Check sheet for the drawn part. Datum: minimum x, y, z corner. Units: mm. A direction names the side the tool comes from. Round coordinates to 2 decimals unless told otherwise and drop trailing zeros. Write each loop counter-clockwise with the first axis right and the second up, starting at its lowest first coordinate (ties: lowest second). Pieces come first, ordered by that corner, then holes. Notation, with made-up numbers: (17.5, -6) -> (46.5, -6) arc R15 ccw to (46.5, 6) -> close; hole circle Ø3 at (85, 4.25). An arc over 180 degrees is marked (long way). Use a Markdown table: item, result.
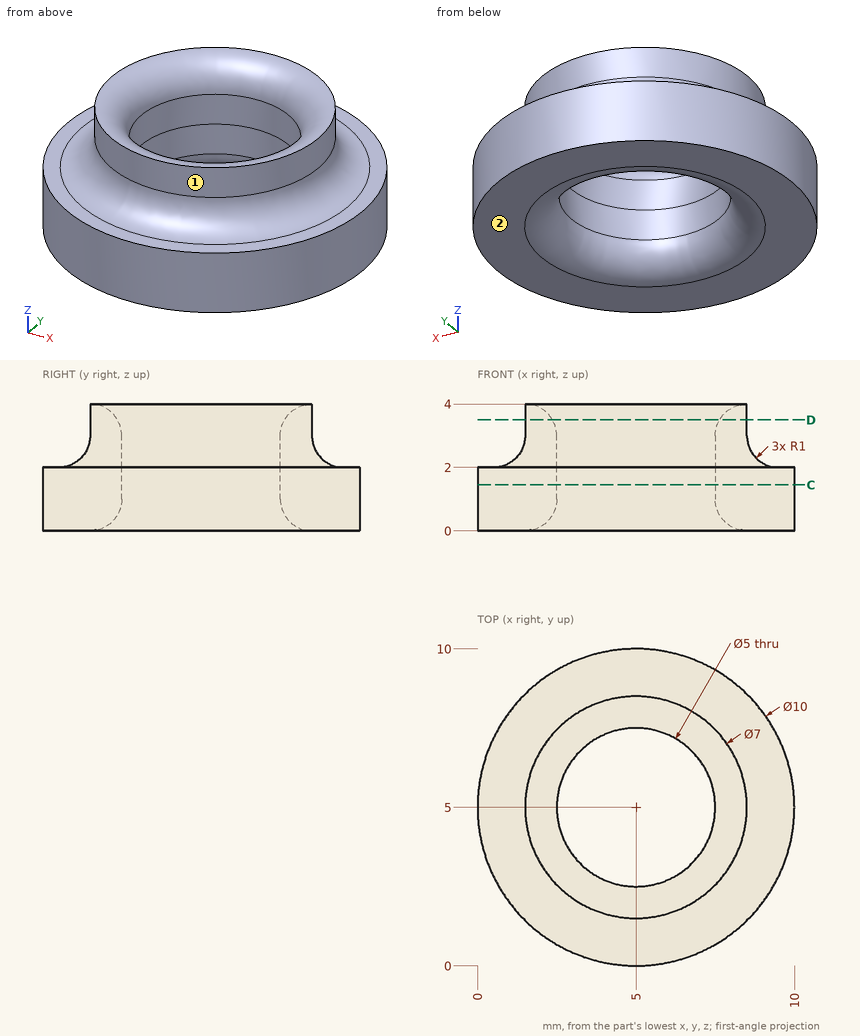
(1) Thickness scan on line 1 (Y direction, x = 5, z = 1.4); line 2 (Y direction, x = 3, z = 0.65); line 3 (X direction, y = 7.25, z = 2.65). Record the ranges inside material, lowest first.
A:
| item | result |
|---|---|
| line 1 | y = 0 to 2.5, 7.5 to 10 |
| line 2 | y = 0.42 to 3.4, 6.6 to 9.58 |
| line 3 | x = 2.24 to 3.91, 6.09 to 7.76 |
(2) Section check D-D on z = 3.5. Record the cut outline in (x, y), plus the area to 3 significant figures.
A:
| item | result |
|---|---|
| outline | circle Ø7 at (5, 5); hole circle Ø5.27 at (5, 5) |
| area | 16.7 mm2 |
(3) Section check C-C on z = 1.45. Record the cut outline in (x, y).
A:
| item | result |
|---|---|
| outline | circle Ø10 at (5, 5); hole circle Ø5 at (5, 5) |
(4) Access from +Z, -Z, +X, -X, +Y, -Y to the whole of each face (thin tool, end or side, straight path). Record for the marked faces 1 and 2.
A:
| item | result |
|---|---|
| face 1 | +Z |
| face 2 | -Z, +X, -X, +Y, -Y |
(5) Gauge pin test, flat ends, axial feed: pin 1 Ø4.5 at (x, y) = (5, 5) entering from -Z; pin 2 Ø1.5 at (x, z) = (3.5, 3) entering from +Y; pin 3 Ø2 at (y, z) = (6.5, 2) entering from +X (3 decimals). Record the tip position at first contact, or that the pin passes through.
A:
| item | result |
|---|---|
| pin 1 | passes through |
| pin 2 | stops at y = 8.58 |
| pin 3 | stops at x = 9.975 |
